Geometry: final body of the model. Coordinates: model frame, mm. A direction names the side the tool comes from. Round coordinates to 2 decimals unless told otherwise and drop trailing zeros. Loops run counter-clockwise (first coordinate to the right, second up) from the corner with the lowest first, then second, coordinate; pieces in that order, holes last. Notation, with made-up numbers: (87, 21.5) - (110, 21.5) arc R15 ccw to (110, 33.5) - close; hole circle Ø7 at (73.5, -30.5). An arc over 180 degrees is marked (long way). Return JSON: item names as keys, results as strings. Group by question number.
1. Draft query along Z for faces 1 (the face through (-1.479, -174.674, 29.465)), 2 (the face through (-1, -192, 0)), 3 (the face through (-20, -168.889, 35)). Return one class per face: +Z half, -Z half, draft (parallel to the pull), parting line (faces both ways), or undercut.
2. Section B-B on y = -182.75. Count the separate pieces of the cut face and the enclosed holes in it, and give its area (3 significant figures).
3. Section A-A on z = 13.5. Return loops of the section in (x, y), and give its area (3 significant figures).
4. Material intervals for probe 1 along X at (y, z) = (-169.5, 9); probe 2 along Z at (x, y) = (-5, -172.25); probe 3 along Z at (x, y) = (-13.5, -177), sorted ascending.
5. First-contact query: pin 1 Ø1.9 at (y, z) = (-171, 35) entering from -X; pin 2 Ø1.5 at (x, y) = (-34.5, -185) entering from +Z; pin 3 Ø4 at (x, z) = (-17.5, 24) entering from -Y. Flat tips, straight axial feed; report the tip coordinate or a pass-through.
6. Set-up query: faces 4 (the face through (-3, -171, 36)), 5 (the face through (-1, -179, 33.489)), 6 (the face through (-38.52, -184.55, 36.55)), 7 (the face through (-20, -179.889, 24)), 8 (the face through (-38.521, -187.664, 10.761)). Return all of +Z, -Z, +X, -X, +Y, -Y with unobstructed straight access to the full face (end or side cutting, diameter ignored); none if empty.
from build123d import *

# Parameters (mm, degrees)
F0_W        = 1
F0_H        = 3.5
F1_DEPTH    = 3
F2_DEPTH    = 20
F4_DEPTH    = 17
F6_T1_DEPTH = 6.9276237231
F6_T3_DEPTH = 6.9276237231


# Not quite as in the source:
# - a fillet or chamfer that OpenCascade refuses, or shapes differently, is made with other operations: its cross-section is extruded or revolved along the edge and cut away or added


with BuildPart() as f1:
    # F0 (on Right) → F1 (new body)
    with BuildSketch(Plane.YZ):
        Polygon((-185.4956659779, 34.4343371689), (-193.88920142, 0), (-190.2867229659, 0), (-184.9662980764, 21.8269531103), (-184.1131562284, 25.3269531103), (-182.1236807397, 33.4887426496), (-178.88920142, 33.4887426496), (-175.6547221004, 33.4887426496), (-173.6652466117, 25.3269531103), (-172.8121047636, 21.8269531103), (-167.4916798742, 0), (-163.88920142, 0), (-172.2827368621, 34.4343371689), (-178.88920142, 34.4343371689), align=None)
        Polygon((-184.8730173458, 36.9887426496), (-185.4956659779, 34.4343371689), (-178.88920142, 34.4343371689), (-172.2827368621, 34.4343371689), (-172.9053854942, 36.9887426496), (-178.88920142, 36.9887426496), align=None)
        Polygon((-184.1131562284, 25.3269531103), (-184.9662980764, 21.8269531103), (-179.88920142, 21.8269531103), (-179.88920142, 25.3269531103), align=None)
        with Locations((-178.38920142, 23.5769531103)):
            Rectangle(F0_W, F0_H)
        with Locations((-179.38920142, 23.5769531103)):
            Rectangle(F0_W, F0_H)
        Polygon((-177.88920142, 21.8269531103), (-172.8121047636, 21.8269531103), (-173.6652466117, 25.3269531103), (-177.88920142, 25.3269531103), align=None)
    extrude(amount=-F1_DEPTH)

    # F0 (on Right) → F2 (join)
    with BuildSketch(Plane.YZ):
        with Locations((-179.38920142, 23.5769531103)):
            Rectangle(F0_W, F0_H)
        with Locations((-178.38920142, 23.5769531103)):
            Rectangle(F0_W, F0_H)
    extrude(amount=-F2_DEPTH)

    # F3 (on face) → F4 (join, through all)
    with BuildSketch(Plane(origin=(-3, 0, 0), x_dir=(0, -1, 0), z_dir=(-1, 0, 0))):
        with BuildLine():
            Line((168.88920142, 34.4301523733), (172.2817167981, 34.4301523733))
            Line((172.2817167981, 34.4301523733), (172.8685340256, 36.8375601227))
            add(Edge.make_bspline(
                [(168.88920142, 35.9301523733), (168.88920142, 36.5362981599), (170.5285389627, 36.7602466997), (172.8685340256, 36.8375601227)],
                knots=[0, 0, 0, 0, 0.2862985804, 0.2862985804, 0.2862985804, 0.2862985804], degree=3))
            Line((168.88920142, 35.9301523733), (168.88920142, 34.4301523733))
        make_face()
        with BuildLine():
            Line((184.9191853663, 36.7993391266), (185.496686042, 34.4301523733))
            Line((185.496686042, 34.4301523733), (188.88920142, 34.4301523733))
            Line((188.88920142, 34.4301523733), (188.88920142, 35.9301523733))
            add(Edge.make_bspline(
                [(184.9191853663, 36.7993391266), (187.2542140028, 36.7124384565), (188.88920142, 36.4941599471), (188.88920142, 35.9301523733)],
                knots=[0.7140815311, 0.7140815311, 0.7140815311, 0.7140815311, 1, 1, 1, 1], degree=3))
        make_face()
        with BuildLine():
            Line((172.2817167981, 34.4301523733), (178.88920142, 34.4301523733))
            Line((178.88920142, 34.4301523733), (185.496686042, 34.4301523733))
            Line((185.496686042, 34.4301523733), (184.9191853663, 36.7993391266))
            add(Edge.make_bspline(
                [(172.8685340256, 36.8375601227), (174.6151730279, 36.895269065), (178.8930025349, 36.8472471546), (183.1708320419, 36.8644060269), (184.9191853663, 36.7993391266)],
                knots=[0.2862985804, 0.2862985804, 0.2862985804, 0.2862985804, 0.5, 0.7140815311, 0.7140815311, 0.7140815311, 0.7140815311], degree=3))
            Line((172.8685340256, 36.8375601227), (172.2817167981, 34.4301523733))
        make_face()
    extrude(amount=F4_DEPTH)

    # F5: F1 across face


with BuildPart() as f1_1:
    add(f1.part)
    add(f1.part.mirror(Plane(origin=(-20, -178.8538492179, 35.6039729667), x_dir=(0, -1, 0), z_dir=(-1, 0, 0))))

    # F6: fillet of radius 2 on 4 edges, made by hand

    # F6_s2 → F6_t1 (cut)
    with BuildSketch(Plane.YZ.offset(-3)):
        with BuildLine():
            ThreePointArc((-185.2450745508, 35.4623842598), (-184.5374266336, 36.561524138), (-183.3019678566, 36.9887426496))
            Line((-183.3019678566, 36.9887426496), (-184.8730173458, 36.9887426496))
            Line((-184.8730173458, 36.9887426496), (-185.2450745508, 35.4623842598))
        make_face()
        with BuildLine():
            ThreePointArc((-172.5333282893, 35.4623842598), (-173.2409762064, 36.561524138), (-174.4764349835, 36.9887426496))
            Line((-174.4764349835, 36.9887426496), (-172.9053854942, 36.9887426496))
            Line((-172.9053854942, 36.9887426496), (-172.5333282893, 35.4623842598))
        make_face()
    extrude(amount=F6_T1_DEPTH, mode=Mode.SUBTRACT)

    # F6_s4 → F6_t3 (cut)
    with BuildSketch(Plane.YZ.offset(-43.9276237231)):
        with BuildLine():
            ThreePointArc((-185.2450745508, 35.4623842598), (-184.5374266336, 36.561524138), (-183.3019678566, 36.9887426496))
            Line((-183.3019678566, 36.9887426496), (-184.8730173458, 36.9887426496))
            Line((-184.8730173458, 36.9887426496), (-185.2450745508, 35.4623842598))
        make_face()
        with BuildLine():
            ThreePointArc((-172.5333282893, 35.4623842598), (-173.2409762064, 36.561524138), (-174.4764349835, 36.9887426496))
            Line((-174.4764349835, 36.9887426496), (-172.9053854942, 36.9887426496))
            Line((-172.9053854942, 36.9887426496), (-172.5333282893, 35.4623842598))
        make_face()
    extrude(amount=F6_T3_DEPTH, mode=Mode.SUBTRACT)


solid = f1_1.part
Taken from the geometry:
{
 "1": {"face 1": "undercut", "face 2": "-Z half", "face 3": "draft"},
 "2": {"separate pieces": "3", "enclosed holes": "0", "area": "140 mm2"},
 "3": {"outline": "(-40, -190.6) - (-37, -190.6) - (-37, -187) - (-40, -187) - close; (-40, -170.78) - (-37, -170.78) - (-37, -167.18) - (-40, -167.18) - close; (-3, -190.6) - (0, -190.6) - (0, -187) - (-3, -187) - close; (-3, -170.78) - (0, -170.78) - (0, -167.18) - (-3, -167.18) - close", "area": "43.2 mm2"},
 "4": {"probe 1": "-40 to -37, -3 to 0", "probe 2": "34.43 to 36.81", "probe 3": "34.43 to 36.87"},
 "5": {"pin 1": "x = -37", "pin 2": "z = 36.82", "pin 3": "y = -179.89"},
 "6": {"face 4": "+Z, +X, +Y", "face 5": "+X, -X", "face 6": "+Z, -X, -Y", "face 7": "-Z, -Y", "face 8": "-Z, +X, -X"}
}
